CAD build for the part. Positions are in the model's coordinates, mm. A direction names the side the tool comes from. Round coordinates to 2 decimals unless told otherwise and drop trailing zeros. Loops run counter-clockwise (first coordinate to the right, second up) from the corner with the lowest first, then second, coordinate; pieces in that order, holes last. Notation, with made-up numbers: (60.5, -20.5) - (78.5, -20.5) arc R14 cw to (78.5, -13.5) - close; hole circle Ø1 at (-25, -26). An arc over 180 degrees is marked (long way). One line per question, with ' | ' between items.
```python
from build123d import *

# Parameters (mm, degrees)
F0_R     = 11
F1_DEPTH = 80
F2_R     = 11
F3_DEPTH = 5


with BuildPart() as f1:
    # F0 (on Front) → F1 (new body)
    with BuildSketch(Plane.XZ):
        Circle(F0_R)
        with BuildLine():
            Line((-2.5, 7.5), (2.5, 7.5))
            ThreePointArc((2.5, 7.5), (6.035534, 6.035534), (7.5, 2.5))
            Line((7.5, 2.5), (7.5, -2.5))
            ThreePointArc((7.5, -2.5), (6.035534, -6.035534), (2.5, -7.5))
            Line((2.5, -7.5), (-2.5, -7.5))
            ThreePointArc((-2.5, -7.5), (-6.035534, -6.035534), (-7.5, -2.5))
            Line((-7.5, -2.5), (-7.5, 2.5))
            ThreePointArc((-7.5, 2.5), (-6.035534, 6.035534), (-2.5, 7.5))
        make_face(mode=Mode.SUBTRACT)
    extrude(amount=F1_DEPTH)

    # F2 (on face) → F3 (join)
    with BuildSketch(Plane(origin=(0, 0, 0), x_dir=(-1, 0, 0), z_dir=(0, 1, 0))):
        Circle(F2_R)
    extrude(amount=F3_DEPTH)


solid = f1.part
```
(1) Cut at D-D, the plane z = 8.5. Write the cut outline in (x, y), then the cut area to 3 significant figures.
Results found:
outline: (-6.98, -80) - (6.98, -80) - (6.98, 5) - (-6.98, 5) - close | area: 1,190 mm²
(2) Cut at B-B, the plane x = 0. Write the cut outline in (y, z).
Results found:
outline: (-80, -11) - (5, -11) - (5, 11) - (-80, 11) - (-80, 7.5) - (0, 7.5) - (0, -7.5) - (-80, -7.5) - close
(3) Two-plate mould, pull along X, no slides. Class faces 1 (the face through (6.07, -39.44, -6)), 2 (the face through (0, 5, 0)): released by +X, released by -X, zero draft, split by the parting line, or undercut.
Results found:
face 1: undercut | face 2: zero draft
(4) Cut at A-A, the plane y = -53.5. Write the cut outline in (x, z), then the cut area to 3 significant figures.
Results found:
outline: circle Ø22 at (0, 0); hole (-7.5, -2.5) arc R5 ccw to (-2.5, -7.5) - (2.5, -7.5) arc R5 ccw to (7.5, -2.5) - (7.5, 2.5) arc R5 ccw to (2.5, 7.5) - (-2.5, 7.5) arc R5 ccw to (-7.5, 2.5) - close | area: 177 mm²
(5) Drop flat-ended pins along their axis: P1, Ø5, axis at x = -8.5, y = -68, coming from the -Z side; P2, Ø2.5, axis at x = -0.5, y = -42.5, coming from the -Z side; P3, Ø6, axis at y = -61, z = -7.5, coming from the -X side; P4, Ø5, axis at y = -30.5, z = 3, coming from the -X side. Give the stop position or say it passes through.
Results found:
P1: stops at z = -9.22 | P2: stops at z = -11 | P3: stops at x = -10.04 | P4: stops at x = -10.99
(6) Probe L1, parallel to Z at x = -0.25, y = -32; L2, parallel to Y at x = -5.75, z = 0; L3, parallel to Z at x = -5.5, y = -65. List the from-to ranges inside material, lowest first.
Results found:
L1: z = -11 to -7.5, 7.5 to 11 | L2: y = 0 to 5 | L3: z = -9.53 to -6.5, 6.5 to 9.53
(7) Tool access for faces 3 (the face through (0, -39, -7.5)), 4 (the face through (8, -80, 0)): list every direction of +Z, -Z, +X, -X, +Y, -Y with a clear straight run to the whole face (end or side of a thin tool).
Results found:
face 3: -Y | face 4: +Z, -Z, +X, -X, -Y
(8) Cut at C-C, the plane z = 0. Write the cut outline in (x, y), then the cut area to 3 significant figures.
Results found:
outline: (-11, -80) - (-7.5, -80) - (-7.5, 0) - (7.5, 0) - (7.5, -80) - (11, -80) - (11, 5) - (-11, 5) - close | area: 670 mm²
